Autodesk Inventor part; units mm, degrees
ref_plane "YZ Plane" through (0, 0, 0) normal (1, 0, 0) x (0, 1, 0)
ref_plane "XZ Plane" through (0, 0, 0) normal (0, 1, 0) x (-1, 0, 0)
ref_plane "XY Plane" through (0, 0, 0) normal (0, 0, 1) x (1, 0, 0)
sketch "Sketch1" plane through (0, 0, 0) normal (0, 0, 1) x (1, 0, 0)
  circle A0 centre (0, 0) radius 3.9688
  dimension "d0" = 7.9375
extrude "Extrusion1" add sketch "Sketch1" along normal blind 28.6957
hole "Hole1" at (0, 0, 0) direction (0, 0, 1) diameter 4.318 end through all
sketch "Sketch2" plane through (0, 0, 28.6957) normal (0, 0, 1) x (1, 0, 0)
  circle A0 centre (0, 0) radius 3.9687
  circle A1 centre (0, 0) radius 6.35
  dimension "d10" = 12.7
extrude "Extrusion2" add sketch "Sketch2" against normal blind 1.5875
fillet "Fillet1" radius 3.175 1 edges at (-3.9687, 0, 27.1082)
properties part number "Supporting Plate Standoff Thin"
The model under review builds one solid part; all positions refer to its coordinate system, in mm. A direction names the side the tool comes from. Round coordinates to 2 decimals unless told otherwise and drop trailing zeros. Loops run counter-clockwise (first coordinate to the right, second up) from the corner with the lowest first, then second, coordinate; pieces in that order, holes last. Notation, with made-up numbers: (12.25, 73.25) -> (55.25, 73.25) arc R18 cw to (55.25, 94.25) -> close; hole circle Ø3 at (13, -13.75). An arc over 180 degrees is marked (long way). Answer as a JSON object with one key per item and string values. Group by question number.
1) We need section A-A on x = 0. Write out the cut boundary in (y, z) (3 decimals), then the cut area to 3 significant figures.
2) For faces 4 (the face through (3.666, 1.52, 11.849)), 5 (the face through (3, 0, 28.696)), list the 3-axis set-ups (+Z, -Z, +X, -X, +Y, -Y) from which the entire face can be reached by the end or side of a thin tool; tool diameter is ignored.
3) Mouldability with a two-part tool opening along Y and no side actions: class faces 1 (the face through (2, -2, 0)), 2 (the face through (-1.38, -6.2, 27.91)), 3 (the face through (-2.14, -0.28, 14.55)) as released by +Y, released by -Y, zero draft, split by the parting line, or undercut.
4) For line 1 (Y direction, x = 0, z = 12.25); line 2 (X direction, y = -1, z = 20.75); line 3 (Y direction, x = -0.5, z = 14), list the stretches that pass through material, from the lowest coordinate up. Write a range as [from, to].
5) We need section C-C on z = 16.75. Write out the cut boundary in (x, y).
6) For pin 1 Ø1 at (y, z) = (-3.5, 4.5) entering from -X, flat-tipped, find the tip position at first contact; note if it passes through.
Result set:
{
 "1": {"outline": "(-6.35, 27.108) arc R3.175 cw to (-3.969, 24.034) -> (-3.969, 0) -> (-2.159, 0) -> (-2.159, 28.696) -> (-6.35, 28.696) -> close; (2.159, 0) -> (3.969, 0) -> (3.969, 24.034) arc R3.175 cw to (6.35, 27.108) -> (6.35, 28.696) -> (2.159, 28.696) -> close", "area": "115 mm²"},
 "2": {"face 4": "-Z", "face 5": "+Z, +X, -X, +Y, -Y"},
 "3": {"face 1": "zero draft", "face 2": "split by the parting line", "face 3": "undercut"},
 "4": {"line 1": "[-3.97, -2.16], [2.16, 3.97]", "line 2": "[-3.84, -1.91], [1.91, 3.84]", "line 3": "[-3.94, -2.1], [2.1, 3.94]"},
 "5": {"outline": "circle Ø7.94 at (0, 0); hole circle Ø4.32 at (0, 0)"},
 "6": {"pin 1": "x = -2.6"}
}
